```python
from build123d import *

# Parameters (mm, degrees)
F0_R     = 12.5
F1_DEPTH = 10


with BuildPart() as f1:
    # F0 (on Front) → F1 (new body)
    with BuildSketch(Plane.XZ):
        Polygon((105.25, -35.124361), (140, -35), (140, -25), (130, -25), (130, -15), (139.429527, -15), (139.429527, -5), (130, -5), (130, 5), (139.429527, 5), (139.429527, 15), (130, 15), (130, 25), (140, 25), (140, 35), (105.25, 35.124361), (105.25, 25.124361), (70, 25.124361), (70, 35.124361), (35.25, 35.124361), (35.25, 25.124361), (0, 25.124361), (-35.25, 25.124361), (-35.25, 35.124361), (-70, 35.124361), (-70, 25.124361), (-105.25, 25.124361), (-105.25, 35.124361), (-140, 35), (-140, 25), (-130, 25), (-130, 15), (-139.429527, 15), (-139.429527, 5), (-130, 5), (-130, -5), (-139.429527, -5), (-139.429527, -15), (-130, -15), (-130, -25), (-140, -25), (-140, -35), (-105.25, -35.124361), (-105.25, -25.124361), (-70, -25.124361), (-70, -35.124361), (-35.25, -35.124361), (-35.25, -25.124361), (0, -25.124361), (35.25, -25.124361), (35.25, -35.124361), (70, -35.124361), (70, -25.124361), (105.25, -25.124361), align=None)
        with Locations((93.097828, -5.217392)):
            Circle(F0_R, mode=Mode.SUBTRACT)
    extrude(amount=F1_DEPTH)


solid = f1.part
```
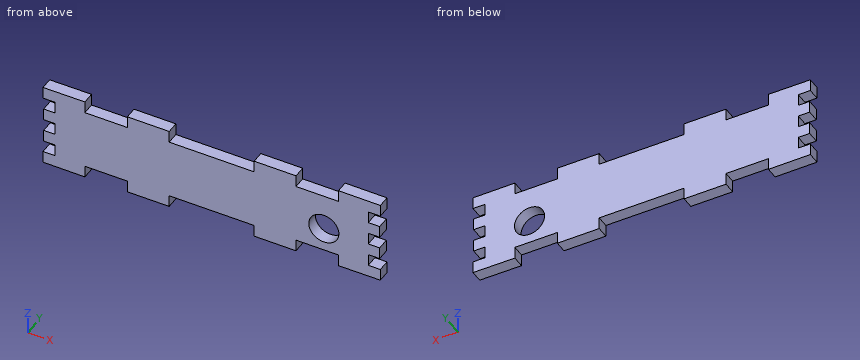
CAD build for the part. Positions are in the model's coordinates, mm. Coordinates: 2 decimals unless noted, no trailing zeros. Loops run counter-clockwise (first coordinate to the right, second up) from the corner with the lowest first, then second, coordinate; pieces in that order, holes last. Notation, with made-up numbers: (83, 51.25) - (99, 51.25) arc R15 cw to (99, 56.25) - close; hole circle Ø2 at (79.25, -6.5). An arc over 180 degrees is marked (long way). Use CSV: the item, a comma, the result in double quotes. Start each with the question number.
Q1. Drop flat-ended pins along their axis: P1, Ø1, axis at x = 28, y = -7.5, coming from the +Z side; P2, Ø3, axis at x = 135.5, y = -6.5, coming from the -Z side; P3, Ø6, axis at x = 84.5, y = -6.5, coming from the -Z side. Give the stop position or say it passes through.
Q2. Cut at C-C, the plane z = 20.5. List the corners of the cut face in (x, y), then the cut area to 3 significant figures.
Q3. Cut at A-A, the plane z = -9. List the corners of the cut face in (x, y).
Q4. Probe probe 1 along X at (y, z) = (-8.75, 25.5); probe 2 along Z at (x, y) = (93.5, -8.25); probe 3 along X at (y, z) = (-0.5, -24). List the from-to ranges inside material, lowest first. Write a range as from..to.
Q5. Cut at B-B, the plane x = 25.5. List the corners of the cut face in (y, z).
Here are the results:
1,P1,"z = 25.12"
1,P2,"z = -35.02"
1,P3,"z = -25.12"
2,outline,"(-130, -10) - (130, -10) - (130, 0) - (-130, 0) - close"
2,area,"2,600 mm2"
3,outline,"(-139.43, -10) - (81.18, -10) - (81.18, 0) - (-139.43, 0) - close; (105.01, -10) - (139.43, -10) - (139.43, 0) - (105.01, 0) - close"
4,probe 1,"-140..-105.25, -70..-35.25, 35.25..70, 105.25..140"
4,probe 2,"-25.12..-17.71, 7.28..25.12"
4,probe 3,"-130..130"
5,outline,"(-10, -25.12) - (0, -25.12) - (0, 25.12) - (-10, 25.12) - close"
